Read the model definition and answer for the solid it produces. Units are mm, in the model's axes. A direction names the side the tool comes from. Give positions to 0.01 mm unless a question says otherwise; leave off trailing zeros. Write each loop counter-clockwise with the first axis right and the second up, starting at its lowest first coordinate (ties: lowest second). Pieces come first, ordered by that corner, then holes. Notation, with made-up numbers: (-33, 24.25) -> (24, 24.25) arc R29 cw to (24, 58.25) -> close; hole circle Ø10 at (-35, -12.5). An arc over 180 degrees is marked (long way). Write item = value, one per line.
from build123d import *

# Parameters (mm, degrees)
BOSS_EXTRUDE1_DEPTH  = 2.4
CHAMFER1_SIZE        = 0.5
BOSS_EXTRUDE2_START  = -52
SKETCH2_W            = 5
SKETCH2_H            = 1.21
BOSS_EXTRUDE2_DEPTH  = 8
BOSS_EXTRUDE3_START  = 14
SKETCH3_W            = 5
SKETCH3_H            = 1.21
BOSS_EXTRUDE3_DEPTH  = 8
BOSS_EXTRUDE4_START  = -52
SKETCH4_W            = 5
SKETCH4_H            = 1.21
BOSS_EXTRUDE4_DEPTH  = 8
BOSS_EXTRUDE5_START  = 14
SKETCH5_W            = 5
SKETCH5_H            = 1.21
BOSS_EXTRUDE5_DEPTH  = 8
BOSS_EXTRUDE6_START  = -44
SKETCH6_W            = 1.5
SKETCH6_H            = 4.01
BOSS_EXTRUDE6_DEPTH  = 58
BOSS_EXTRUDE7_START  = -40
SKETCH7_W            = 4.8
SKETCH7_H            = 18.36
BOSS_EXTRUDE7_DEPTH  = 10
BOSS_EXTRUDE8_START  = 8
SKETCH8_R            = 1
BOSS_EXTRUDE8_DEPTH  = 13.75
BOSS_EXTRUDE9_START  = -53.8
SKETCH9_W            = 7
SKETCH9_H            = 4.01
BOSS_EXTRUDE9_DEPTH  = 1.5
BOSS_EXTRUDE10_START = 24.3
SKETCH10_W           = 7
SKETCH10_H           = 4.01
BOSS_EXTRUDE10_DEPTH = 1.5
BOSS_EXTRUDE11_START = -44
SKETCH11_W           = 1.5
SKETCH11_H           = 4.01
BOSS_EXTRUDE11_DEPTH = 58
BOSS_EXTRUDE12_START = -40
SKETCH12_W           = 4.8
SKETCH12_H           = 18.36
BOSS_EXTRUDE12_DEPTH = 10
BOSS_EXTRUDE13_START = 8
SKETCH13_R           = 1
BOSS_EXTRUDE13_DEPTH = 13.75
BOSS_EXTRUDE14_START = -53.8
SKETCH14_W           = 7
SKETCH14_H           = 4.01
BOSS_EXTRUDE14_DEPTH = 1.5
BOSS_EXTRUDE15_START = 24.3
SKETCH15_W           = 7
SKETCH15_H           = 4.01
BOSS_EXTRUDE15_DEPTH = 1.5
BOSS_EXTRUDE16_START = -1
SKETCH16_R           = 2.1
BOSS_EXTRUDE16_DEPTH = 3.6
BOSS_EXTRUDE17_START = 2.5
SKETCH17_R           = 1.3
BOSS_EXTRUDE17_DEPTH = 1.2
BOSS_EXTRUDE18_START = -1
SKETCH18_R           = 2.1
BOSS_EXTRUDE18_DEPTH = 3.6
BOSS_EXTRUDE19_START = 2.5
SKETCH19_R           = 1.3
BOSS_EXTRUDE19_DEPTH = 1.2
BOSS_EXTRUDE20_START = -1
SKETCH20_R           = 2.1
BOSS_EXTRUDE20_DEPTH = 3.6
BOSS_EXTRUDE21_START = 2.5
SKETCH21_R           = 1.3
BOSS_EXTRUDE21_DEPTH = 1.2
BOSS_EXTRUDE22_START = -1
SKETCH22_R           = 2.1
BOSS_EXTRUDE22_DEPTH = 3.6
BOSS_EXTRUDE23_START = 2.5
SKETCH23_R           = 1.3
BOSS_EXTRUDE23_DEPTH = 1.2
BOSS_EXTRUDE24_START = -54.1
SKETCH24_W           = 4
SKETCH24_H           = 0.9
BOSS_EXTRUDE24_DEPTH = 1


with BuildPart() as part:
    # Sketch1 → Boss-Extrude1 (new body)
    with BuildSketch(Plane(origin=(0, 0, 0), x_dir=(1, 0, 0), z_dir=(0, 1, 0))):
        with BuildLine():
            Line((-23, 54), (23, 54))
            ThreePointArc((23, 54), (25.121320344, 53.121320344), (26, 51))
            Line((26, 51), (26, -23))
            ThreePointArc((26, -23), (25.121320344, -25.121320344), (23, -26))
            Line((23, -26), (-23, -26))
            ThreePointArc((-23, -26), (-25.121320344, -25.121320344), (-26, -23))
            Line((-26, -23), (-26, 51))
            ThreePointArc((-26, 51), (-25.121320344, 53.121320344), (-23, 54))
        make_face()
    extrude(amount=BOSS_EXTRUDE1_DEPTH)

    # Chamfer1
    chamfer1_edges = [part.edges().sort_by_distance(p)[0] for p in [
        (0, 0, 26),
        (-25.121320344, 0, 25.121320344),
        (-26, 0, -14),
        (-25.121320344, 0, -53.121320344),
        (0, 0, -54),
        (25.121320344, 0, -53.121320344),
        (26, 0, -14),
        (25.121320344, 0, 25.121320344),
    ]]
    chamfer(chamfer1_edges, length=CHAMFER1_SIZE)

    # Sketch2 → Boss-Extrude2 (add)
    with BuildSketch(Plane.XY.offset(BOSS_EXTRUDE2_START)):
        with Locations((-23.4, 2.995)):
            Rectangle(SKETCH2_W, SKETCH2_H)
    extrude(amount=BOSS_EXTRUDE2_DEPTH)

    # Sketch3 → Boss-Extrude3 (add)
    with BuildSketch(Plane.XY.offset(BOSS_EXTRUDE3_START)):
        with Locations((-23.4, 2.995)):
            Rectangle(SKETCH3_W, SKETCH3_H)
    extrude(amount=BOSS_EXTRUDE3_DEPTH)

    # Sketch4 → Boss-Extrude4 (add)
    with BuildSketch(Plane.XY.offset(BOSS_EXTRUDE4_START)):
        with Locations((23.4, 2.995)):
            Rectangle(SKETCH4_W, SKETCH4_H)
    extrude(amount=BOSS_EXTRUDE4_DEPTH)

    # Sketch5 → Boss-Extrude5 (add)
    with BuildSketch(Plane.XY.offset(BOSS_EXTRUDE5_START)):
        with Locations((23.4, 2.995)):
            Rectangle(SKETCH5_W, SKETCH5_H)
    extrude(amount=BOSS_EXTRUDE5_DEPTH)

    # Sketch6 → Boss-Extrude6 (add)
    with BuildSketch(Plane.XY.offset(BOSS_EXTRUDE6_START)):
        with Locations((-21.45, 4.395)):
            Rectangle(SKETCH6_W, SKETCH6_H)
    extrude(amount=BOSS_EXTRUDE6_DEPTH)

    # Sketch7 → Boss-Extrude7 (add)
    with BuildSketch(Plane.XY.offset(BOSS_EXTRUDE7_START)):
        with Locations((-23.4, 11.57)):
            Rectangle(SKETCH7_W, SKETCH7_H)
    extrude(amount=BOSS_EXTRUDE7_DEPTH)


with BuildPart() as body_2:
    # Sketch8 → Boss-Extrude8 (new body)
    with BuildSketch(Plane(origin=(0, 0, 0), x_dir=(1, 0, 0), z_dir=(0, 1, 0)).offset(BOSS_EXTRUDE8_START)):
        with Locations(Location((-23.4, 35, 0), (0, 0, 270))):
            Circle(SKETCH8_R)
    extrude(amount=BOSS_EXTRUDE8_DEPTH)


with BuildPart() as part_1:
    add(part.part)

    # Combine1: cut body 2
    add(body_2.part, mode=Mode.SUBTRACT)

    # Sketch9 → Boss-Extrude9 (add)
    with BuildSketch(Plane.XY.offset(BOSS_EXTRUDE9_START)):
        with Locations((-9.5, 4.395)):
            Rectangle(SKETCH9_W, SKETCH9_H)
    extrude(amount=BOSS_EXTRUDE9_DEPTH)

    # Sketch10 → Boss-Extrude10 (add)
    with BuildSketch(Plane.XY.offset(BOSS_EXTRUDE10_START)):
        with Locations((-9.5, 4.395)):
            Rectangle(SKETCH10_W, SKETCH10_H)
    extrude(amount=BOSS_EXTRUDE10_DEPTH)

    # Sketch11 → Boss-Extrude11 (add)
    with BuildSketch(Plane.XY.offset(BOSS_EXTRUDE11_START)):
        with Locations((21.45, 4.395)):
            Rectangle(SKETCH11_W, SKETCH11_H)
    extrude(amount=BOSS_EXTRUDE11_DEPTH)

    # Sketch12 → Boss-Extrude12 (add)
    with BuildSketch(Plane.XY.offset(BOSS_EXTRUDE12_START)):
        with Locations((23.4, 11.57)):
            Rectangle(SKETCH12_W, SKETCH12_H)
    extrude(amount=BOSS_EXTRUDE12_DEPTH)


with BuildPart() as body_2_2:
    # Sketch13 → Boss-Extrude13 (new body)
    with BuildSketch(Plane(origin=(0, 0, 0), x_dir=(1, 0, 0), z_dir=(0, 1, 0)).offset(BOSS_EXTRUDE13_START)):
        with Locations(Location((23.4, 35, 0), (0, 0, 270))):
            Circle(SKETCH13_R)
    extrude(amount=BOSS_EXTRUDE13_DEPTH)


with BuildPart() as part_2:
    add(part_1.part)

    # Combine2: cut body 2 2
    add(body_2_2.part, mode=Mode.SUBTRACT)

    # Sketch14 → Boss-Extrude14 (add)
    with BuildSketch(Plane.XY.offset(BOSS_EXTRUDE14_START)):
        with Locations((9.5, 4.395)):
            Rectangle(SKETCH14_W, SKETCH14_H)
    extrude(amount=BOSS_EXTRUDE14_DEPTH)

    # Sketch15 → Boss-Extrude15 (add)
    with BuildSketch(Plane.XY.offset(BOSS_EXTRUDE15_START)):
        with Locations((9.5, 4.395)):
            Rectangle(SKETCH15_W, SKETCH15_H)
    extrude(amount=BOSS_EXTRUDE15_DEPTH)


with BuildPart() as body_2_3:
    # Sketch16 → Boss-Extrude16 (new body)
    with BuildSketch(Plane(origin=(0, 0, 0), x_dir=(1, 0, 0), z_dir=(0, 1, 0)).offset(BOSS_EXTRUDE16_START)):
        with Locations(Location((-23.4, 48, 0), (0, 0, 270))):
            Circle(SKETCH16_R)
    extrude(amount=BOSS_EXTRUDE16_DEPTH)


with BuildPart() as part_3:
    add(part_2.part)

    # Combine3: cut body 2 3
    add(body_2_3.part, mode=Mode.SUBTRACT)


with BuildPart() as body_2_4:
    # Sketch17 → Boss-Extrude17 (new body)
    with BuildSketch(Plane(origin=(0, 0, 0), x_dir=(1, 0, 0), z_dir=(0, 1, 0)).offset(BOSS_EXTRUDE17_START)):
        with Locations(Location((-23.4, 48, 0), (0, 0, 270))):
            Circle(SKETCH17_R)
    extrude(amount=BOSS_EXTRUDE17_DEPTH)


with BuildPart() as part_4:
    add(part_3.part)

    # Combine4: cut body 2 4
    add(body_2_4.part, mode=Mode.SUBTRACT)


with BuildPart() as body_2_5:
    # Sketch18 → Boss-Extrude18 (new body)
    with BuildSketch(Plane(origin=(0, 0, 0), x_dir=(1, 0, 0), z_dir=(0, 1, 0)).offset(BOSS_EXTRUDE18_START)):
        with Locations(Location((-23.4, -18, 0), (0, 0, 270))):
            Circle(SKETCH18_R)
    extrude(amount=BOSS_EXTRUDE18_DEPTH)


with BuildPart() as part_5:
    add(part_4.part)

    # Combine5: cut body 2 5
    add(body_2_5.part, mode=Mode.SUBTRACT)


with BuildPart() as body_2_6:
    # Sketch19 → Boss-Extrude19 (new body)
    with BuildSketch(Plane(origin=(0, 0, 0), x_dir=(1, 0, 0), z_dir=(0, 1, 0)).offset(BOSS_EXTRUDE19_START)):
        with Locations(Location((-23.4, -18, 0), (0, 0, 270))):
            Circle(SKETCH19_R)
    extrude(amount=BOSS_EXTRUDE19_DEPTH)


with BuildPart() as part_6:
    add(part_5.part)

    # Combine6: cut body 2 6
    add(body_2_6.part, mode=Mode.SUBTRACT)


with BuildPart() as body_2_7:
    # Sketch20 → Boss-Extrude20 (new body)
    with BuildSketch(Plane(origin=(0, 0, 0), x_dir=(1, 0, 0), z_dir=(0, 1, 0)).offset(BOSS_EXTRUDE20_START)):
        with Locations(Location((23.4, 48, 0), (0, 0, 270))):
            Circle(SKETCH20_R)
    extrude(amount=BOSS_EXTRUDE20_DEPTH)


with BuildPart() as part_7:
    add(part_6.part)

    # Combine7: cut body 2 7
    add(body_2_7.part, mode=Mode.SUBTRACT)


with BuildPart() as body_2_8:
    # Sketch21 → Boss-Extrude21 (new body)
    with BuildSketch(Plane(origin=(0, 0, 0), x_dir=(1, 0, 0), z_dir=(0, 1, 0)).offset(BOSS_EXTRUDE21_START)):
        with Locations(Location((23.4, 48, 0), (0, 0, 270))):
            Circle(SKETCH21_R)
    extrude(amount=BOSS_EXTRUDE21_DEPTH)


with BuildPart() as part_8:
    add(part_7.part)

    # Combine8: cut body 2 8
    add(body_2_8.part, mode=Mode.SUBTRACT)


with BuildPart() as body_2_9:
    # Sketch22 → Boss-Extrude22 (new body)
    with BuildSketch(Plane(origin=(0, 0, 0), x_dir=(1, 0, 0), z_dir=(0, 1, 0)).offset(BOSS_EXTRUDE22_START)):
        with Locations(Location((23.4, -18, 0), (0, 0, 270))):
            Circle(SKETCH22_R)
    extrude(amount=BOSS_EXTRUDE22_DEPTH)


with BuildPart() as part_9:
    add(part_8.part)

    # Combine9: cut body 2 9
    add(body_2_9.part, mode=Mode.SUBTRACT)


with BuildPart() as body_2_10:
    # Sketch23 → Boss-Extrude23 (new body)
    with BuildSketch(Plane(origin=(0, 0, 0), x_dir=(1, 0, 0), z_dir=(0, 1, 0)).offset(BOSS_EXTRUDE23_START)):
        with Locations(Location((23.4, -18, 0), (0, 0, 270))):
            Circle(SKETCH23_R)
    extrude(amount=BOSS_EXTRUDE23_DEPTH)


with BuildPart() as part_10:
    add(part_9.part)

    # Combine10: cut body 2 10
    add(body_2_10.part, mode=Mode.SUBTRACT)


with BuildPart() as body_2_11:
    # Sketch24 → Boss-Extrude24 (new body)
    with BuildSketch(Plane.XY.offset(BOSS_EXTRUDE24_START)):
        with Locations((0, 0.35)):
            Rectangle(SKETCH24_W, SKETCH24_H)
    extrude(amount=BOSS_EXTRUDE24_DEPTH)


with BuildPart() as part_11:
    add(part_10.part)

    # Combine11: cut body 2 11
    add(body_2_11.part, mode=Mode.SUBTRACT)


solid = part_11.part
(1) The part is cut by section B-B on y = 4.5. Count the separate pieces of the cut face and the enclosed holes in it, plus the area to 3 significant figures.
Checks:
separate_pieces = 6
enclosed_holes = 0
area = 288 mm²
(2) Given P1, Ø15.5, axis at x = -1.5, z = -33.5, coming from the +Y side; P2, Ø4, axis at x = 23.4, z = -48, coming from the +Y side; P3, Ø4, axis at x = -14.5, y = 8.5, coming from the -Z side; P4, Ø1, axis at x = 4.5, z = -19.5, coming from the -Y side, each flat-ended and moving along its own axis, determine where each tip first touches the part or whether it passes through.
Checks:
P1 = 2.4
P2 = 3.6
P3 = through
P4 = 0
(3) The part is cut by section D-D on x = -1. Determine the outline of the cut face in (y, z), plus the area to 3 significant figures.
Checks:
outline = (0, -53.1) -> (0.8, -53.1) -> (0.8, -54) -> (2.4, -54) -> (2.4, 26) -> (0.5, 26) -> (0, 25.5) -> close
area = 191 mm²
(4) Consider L1, parallel to Z at x = -23.4, y = 3.25; L2, parallel to X at y = 0.95, z = 18; L3, parallel to X at y = 17, z = -35. Determine where each line is inside the solid, lowest interval first.
Checks:
L1 = -52 to -49.3, -46.7 to -44, -40 to -30, 14 to 16.7, 19.3 to 22
L2 = -26 to -25.5, -21.3 to 21.3, 25.5 to 26
L3 = -25.8 to -24.4, -22.4 to -21, 21 to 22.4, 24.4 to 25.8
(5) The part is cut by section A-A on y = 17.25. Determine the outline of the cut face in (x, z), plus the area to 3 significant figures.
Checks:
outline = (-25.8, -40) -> (-21, -40) -> (-21, -30) -> (-25.8, -30) -> close; (21, -40) -> (25.8, -40) -> (25.8, -30) -> (21, -30) -> close; hole circle Ø2 at (-23.4, -35); hole circle Ø2 at (23.4, -35)
area = 89.7 mm²
(6) The part is cut by section C-C on z = -37. Determine the outline of the cut face in (x, y).
Checks:
outline = (-26, 0.5) -> (-25.5, 0) -> (25.5, 0) -> (26, 0.5) -> (26, 2.4) -> (25.8, 2.4) -> (25.8, 20.75) -> (21, 20.75) -> (21, 6.4) -> (20.7, 6.4) -> (20.7, 2.4) -> (-20.7, 2.4) -> (-20.7, 6.4) -> (-21, 6.4) -> (-21, 20.75) -> (-25.8, 20.75) -> (-25.8, 2.4) -> (-26, 2.4) -> close
(7) For a pull along X with two mould halves and no side action, classify faces 5 (the flat face through (-22.2, 4, -8)), 6 (the flat face through (-6, 4, 25)), 7 (the flat face through (22, 3.6, 19)), 8 (the flat face through (13, 4, 25)) as released by +X, released by -X, zero draft, split by the parting line, or undercut.
Checks:
face_5 = released by -X
face_6 = undercut
face_7 = zero draft
face_8 = released by +X
(8) A tool of negligible diameter and unlimited length cuts with its end or side. For faces 1 (the flat face through (-10, 4, -53.8)), 2 (the cylindrical face through (-23.1, 14.286, -34.046)), 3 (the flat face through (-21, 13, -35)), 4 (the flat face through (-22, 2.6, -47)), from which of +Z, -Z, +X, -X, +Y, -Y can it reach the whole face along a straight path? Write none if from no direction.
Checks:
face_1 = -Z, +X, -X, +Y
face_2 = +Y
face_3 = +Z, -Z, +Y
face_4 = -Y
